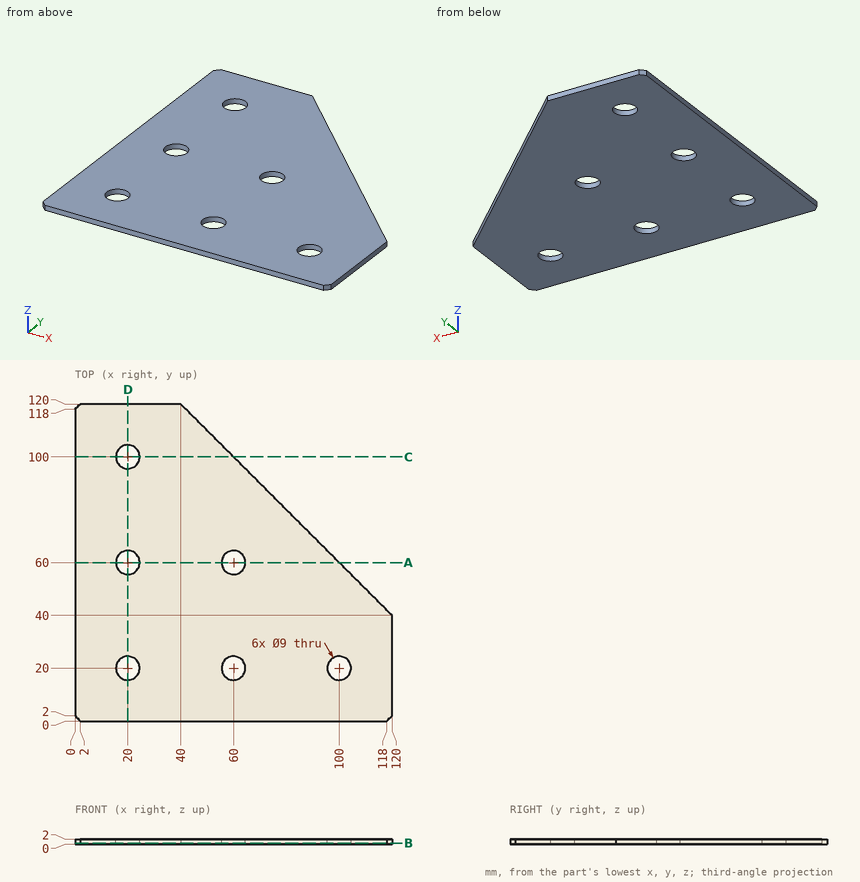
Check sheet for the drawn part. Datum: minimum x, y, z corner. Units: mm. Give positions to 0.01 mm unless a question says otherwise; leave off trailing zeros. Loops run counter-clockwise (first coordinate to the right, second up) from the corner with the lowest first, then second, coordinate; pieces in that order, holes last.
1) Sectioned sample at B-B, the plane z = 0.45. Enter the section's corners in (x, y).
2) Sectioned sample at A-A, the plane y = 60. Enter the section's corners in (x, z), then the cut area to 3 significant figures.
3) Depth check by flat-ended pin: pin 1 Ø8 at (x, y) = (60, 60) entering from -Z; pin 2 Ø1 at (y, z) = (76.5, 1) entering from +X. Enter the tip coordinate at first touch or a pass-through.
4) Sectioned sample at D-D, the plane x = 20. Enter the section's corners in (y, z).
5) Thickness scan on line 1 along X through (y, z) = (20, 1.25); line 2 along X through (y, z) = (60, 0.7). Record the ranges inside material, lowest first.
6) Sectioned sample at C-C, the plane y = 100. Enter the section's corners in (x, z), then the cut area to 3 significant figures.
Answers:
1. outline: (0, 2) - (2, 0) - (118, 0) - (120, 2) - (120, 40) - (40, 120) - (2, 120) - (0, 118) - close; hole circle Ø9 at (20, 20); hole circle Ø9 at (20, 60); hole circle Ø9 at (20, 100); hole circle Ø9 at (60, 20); hole circle Ø9 at (60, 60); hole circle Ø9 at (100, 20)
2. outline: (0, 0) - (15.5, 0) - (15.5, 2) - (0, 2) - close; (24.5, 0) - (55.5, 0) - (55.5, 2) - (24.5, 2) - close; (64.5, 0) - (100, 0) - (100, 2) - (64.5, 2) - close
2. area: 164 mm2
3. pin 1: passes through
3. pin 2: stops at x = 84
4. outline: (0, 0) - (15.5, 0) - (15.5, 2) - (0, 2) - close; (24.5, 0) - (55.5, 0) - (55.5, 2) - (24.5, 2) - close; (64.5, 0) - (95.5, 0) - (95.5, 2) - (64.5, 2) - close; (104.5, 0) - (120, 0) - (120, 2) - (104.5, 2) - close
5. line 1: x = 0 to 15.5, 24.5 to 55.5, 64.5 to 95.5, 104.5 to 120
5. line 2: x = 0 to 15.5, 24.5 to 55.5, 64.5 to 100
6. outline: (0, 0) - (15.5, 0) - (15.5, 2) - (0, 2) - close; (24.5, 0) - (60, 0) - (60, 2) - (24.5, 2) - close
6. area: 102 mm2
